```python
from build123d import *

# Parameters (mm, degrees)
SKETCH_1_W      = 13.9
SKETCH_1_H      = 13.9
EXTRUDE_1_DEPTH = 5.5
FILLET_1_R      = 1


with BuildPart() as part:
    # Эскиз1 → Бобышка-Вытянуть1 (new body)
    with BuildSketch(Plane.XY):
        Rectangle(SKETCH_1_W, SKETCH_1_H)
    extrude(amount=EXTRUDE_1_DEPTH)

    # Эскиз3 → Отверстие обработанное метчиком M81 (revolve, cut)
    with BuildSketch(Plane(origin=(0, 0, 5.5), x_dir=(0, -1, 0), z_dir=(1, 0, 0))):
        Polygon((0, 0), (0, 5.5), (4.025, 5.5), (3.4, 4.875), (3.4, 0.625), (4.025, 0), align=None)
    revolve(axis=Axis((0, 0, 11.85), (0, 0, -1)), mode=Mode.SUBTRACT)

    # Скругление1
    fillet_1_edges = [part.edges().sort_by_distance(p)[0] for p in [
        (6.95, -6.95, 2.75),
        (-6.95, -6.95, 2.75),
        (-6.95, 6.95, 2.75),
        (6.95, 6.95, 2.75),
    ]]
    fillet(fillet_1_edges, radius=FILLET_1_R)


solid = part.part
```
Work out the finished part from the listing and answer in its coordinate system (mm). Coordinates: 2 decimals unless noted, no trailing zeros. Loops run counter-clockwise (first coordinate to the right, second up) from the corner with the lowest first, then second, coordinate; pieces in that order, holes last. Notation, with made-up numbers: (0.25, 15) -> (12.25, 15) arc R37 ccw to (12.25, 52) -> close; hole circle Ø3 at (78, 14.5). An arc over 180 degrees is marked (long way). Answer as CSV lines item,"result".
Q1. The part is cut by section A-A on x = 0. Write down the section's boundary in (y, z) (3 decimals), and give its area (3 significant figures).
Findings:
outline,"(-6.95, 0) -> (-4.025, 0) -> (-3.4, 0.625) -> (-3.4, 4.875) -> (-4.025, 5.5) -> (-6.95, 5.5) -> close; (3.4, 0.625) -> (4.025, 0) -> (6.95, 0) -> (6.95, 5.5) -> (4.025, 5.5) -> (3.4, 4.875) -> close"
area,"38.3 mm²"
Q2. For a pull along Y with two mould halves and no side action, classify faces 1 (the face through (-6.665, 6.649, 2.788)), 2 (the face through (3.32, 0.74, 2.78)), 3 (the face through (-6.665, -6.649, 2.788)), 4 (the face through (-3, -3, 5.5)) as +Y half, -Y half, draft (parallel to the pull), parting line (faces both ways), or undercut.
Findings:
face 1,"+Y half"
face 2,"undercut"
face 3,"-Y half"
face 4,"draft"
Q3. Find the intervals of material crossed by probe 1 along X at (y, z) = (0, 1.75); probe 2 along Y at (x, z) = (-2.25, 4.9), in increasing order.
Findings:
probe 1,"x = -6.95 to -3.4, 3.4 to 6.95"
probe 2,"y = -6.95 to -2.58, 2.58 to 6.95"
Q4. This flat-tipped pin is pushed along its axis until it touches: pin 1 (1 mm diameter, centred on x = -5.5, y = -1, fed in from -Z). Where does it stop, or does it pass through?
Findings:
pin 1,"stops at z = 0"
Q5. The part is cut by section B-B on z = 1.9. Write down the section's boundary in (x, y).
Findings:
outline,"(-6.95, -5.95) arc R1 ccw to (-5.95, -6.95) -> (5.95, -6.95) arc R1 ccw to (6.95, -5.95) -> (6.95, 5.95) arc R1 ccw to (5.95, 6.95) -> (-5.95, 6.95) arc R1 ccw to (-6.95, 5.95) -> close; hole circle Ø6.8 at (0, 0)"
